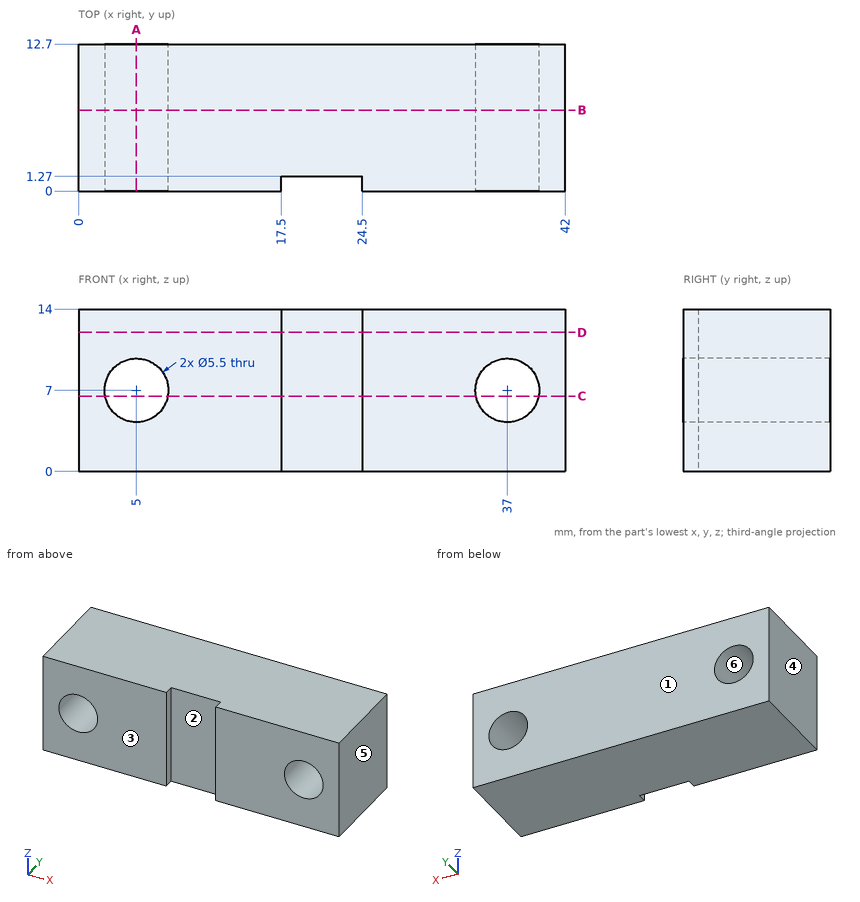
Could you check a few things on this drawing? It's one solid part, dimensions in mm from its lowest x, y, z. A direction names the side the tool comes from. Coordinates: 2 decimals unless noted, no trailing zeros. Order: outer loops, then holes, each group sorted by start corner. A loop starts at its lowest first (then second) coordinate and runs counter-clockwise, first axis right, second up. Notation, with made-up numbers: (63.5, 27) -> (117.5, 27) arc R12 ccw to (117.5, 37) -> close; hole circle Ø10 at (7.25, -21.75). An arc over 180 degrees is marked (long way). One line per item, written item: value. Start each with the question number.
1) Imagine slicing it at D-D on z = 12. List the corners of the cut face in (x, y) for me.
2) If I drill on L1, parallel to X at y = 3, z = 7; L2, parallel to Z at x = 37, y = 5; L3, parallel to X at y = 8.75, z = 6.25, over which ranges is the centre line in solid material (lowest first)? Write a range as [from, to].
3) Which directions (+Z, -Z, +X, -X, +Y, -Y) give clear straight access to the entire face, cutting with the end or side of a thin tool? Please do the marked faces 1 and 2.
4) We'd pull the mould along X, two halves only. Please class the marked faces 3, 4, 5 and 6: +X half, -X half, draft (parallel to the pull), parting line (faces both ways), or undercut.
5) Imagine slicing it at A-A on x = 5. List the corners of the cut face in (y, z) for me.
6) I'm going to push flat-ended pins straight in: pin 1 (3.5 mm diameter, centred on x = 22, z = 8, fed in from -Y); pin 2 (3.5 mm diameter, centred on x = 37, z = 7, fed in from +Y). Where does each tip first touch, or does it pass through?
7) Imagine slicing it at C-C on z = 6.5. List the corners of the cut face in (x, y) for me, plus the area to 3 significant figures.
8) Imagine slicing it at B-B on y = 7. List the corners of the cut face in (x, z) for me.
Answer list:
1. outline: (0, 0) -> (17.5, 0) -> (17.5, 1.27) -> (24.5, 1.27) -> (24.5, 0) -> (42, 0) -> (42, 12.7) -> (0, 12.7) -> close
2. L1: x = [0, 2.25], [7.75, 34.25], [39.75, 42]
2. L2: z = [0, 4.25], [9.75, 14]
2. L3: x = [0, 2.35], [7.65, 34.35], [39.65, 42]
3. face 1: +Z, -Z, +X, -X, +Y
3. face 2: +Z, -Z, -Y
4. face 3: draft
4. face 4: -X half
4. face 5: +X half
4. face 6: undercut
5. outline: (0, 0) -> (12.7, 0) -> (12.7, 4.25) -> (0, 4.25) -> close; (0, 9.75) -> (12.7, 9.75) -> (12.7, 14) -> (0, 14) -> close
6. pin 1: stops at y = 1.27
6. pin 2: passes through
7. outline: (0, 0) -> (2.3, 0) -> (2.3, 12.7) -> (0, 12.7) -> close; (7.7, 0) -> (17.5, 0) -> (17.5, 1.27) -> (24.5, 1.27) -> (24.5, 0) -> (34.3, 0) -> (34.3, 12.7) -> (7.7, 12.7) -> close; (39.7, 0) -> (42, 0) -> (42, 12.7) -> (39.7, 12.7) -> close
7. area: 387 mm2
8. outline: (0, 0) -> (42, 0) -> (42, 14) -> (0, 14) -> close; hole circle Ø5.5 at (5, 7); hole circle Ø5.5 at (37, 7)
